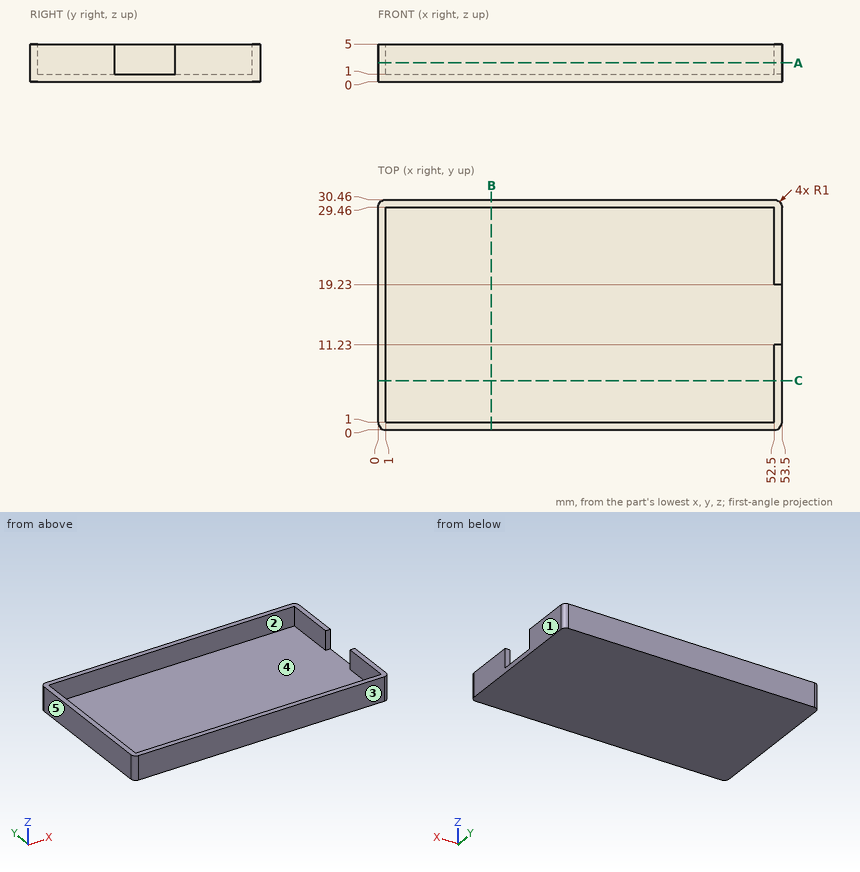
Source: three-view drawing plus pictorial views. Frame: mm from the lowest corner of the part. A direction names the side the tool comes from. Give positions to 0.01 mm unless a question says otherwise; leave off trailing zeros. Loops run counter-clockwise (first coordinate to the right, second up) from the corner with the lowest first, then second, coordinate; pieces in that order, holes last.
1) Section query B-B on x = 15. Return the cut outline in (y, z), and give its area (3 significant figures).
A:
outline: (0, 0) - (30.46, 0) - (30.46, 5) - (29.46, 5) - (29.46, 1) - (1, 1) - (1, 5) - (0, 5) - close
area: 38.5 mm2
2) Mould query, pull axis X, two halves, no side actions, for the marked faces 3, 4 and 5. Classes: released by +X, released by -X, zero draft, split by the parting line, or undercut.
A:
face 3: zero draft
face 4: undercut
face 5: released by -X
3) Reachability of the marked faces 1 and 2 from +Z, -Z, +X, -X, +Y, -Y: full face, straight path, thin tool, end or side. Return the list, or none.
A:
face 1: +Z, -Z, +X, +Y, -Y
face 2: +Z
4) Line query: L1, parallel to X at y = 29, z = 2.4; L2, parallel to Y at x = 50, z = 3.1; L3, parallel to Z at x = 4, y = 8.5. Output: solid intervals per line, ascending.
A:
L1: x = 0 to 1, 52.5 to 53.5
L2: y = 0 to 1, 29.46 to 30.46
L3: z = 0 to 1
5) Contact query for flat-ended pins moving along their axis: pin 1 (3 mm diameter, centred on x = 13.5, y = 24, fed in from +Z); pin 2 (2 mm diameter, centred on y = 5.5, z = 2, fed in from -X). Output: stop coordinate, or through.
A:
pin 1: stops at z = 1
pin 2: stops at x = 0
6) Section query C-C on y = 6.5. Return the cut outline in (x, z), and give its area (3 significant figures).
A:
outline: (0, 0) - (53.5, 0) - (53.5, 5) - (52.5, 5) - (52.5, 1) - (1, 1) - (1, 5) - (0, 5) - close
area: 61.5 mm2
7) Section query A-A on z = 2.5. Return the cut outline in (x, y).
A:
outline: (0, 1) arc R1 ccw to (1, 0) - (52.5, 0) arc R1 ccw to (53.5, 1) - (53.5, 11.23) - (52.5, 11.23) - (52.5, 1) - (1, 1) - (1, 29.46) - (52.5, 29.46) - (52.5, 19.23) - (53.5, 19.23) - (53.5, 29.46) arc R1 ccw to (52.5, 30.46) - (1, 30.46) arc R1 ccw to (0, 29.46) - close
